from build123d import *

# Parameters (mm, degrees)
F0_W     = 1905
F0_H     = 101.6
F1_DEPTH = 25.4
F3_DEPTH = 25.401


with BuildPart() as f1:
    # F0 (on Right) → F1 (new body)
    with BuildSketch(Plane.YZ):
        with Locations((952.5, 50.8)):
            Rectangle(F0_W, F0_H)
    extrude(amount=F1_DEPTH)

    # F2 (on face) → F3 (cut, through all)
    with BuildSketch(Plane.YZ.offset(25.4)):
        with BuildLine():
            ThreePointArc((63.5, 76.2), (59.780256, 85.180256), (50.8, 88.9))
            Line((50.8, 88.9), (50.8, 63.5))
            ThreePointArc((50.8, 63.5), (59.780256, 67.219744), (63.5, 76.2))
        make_face()
        with BuildLine():
            Line((50.8, 63.5), (50.8, 88.9))
            ThreePointArc((50.8, 88.9), (38.1, 76.2), (50.8, 63.5))
        make_face()
        with BuildLine():
            ThreePointArc((1866.9, 76.2), (1863.180256, 85.180256), (1854.2, 88.9))
            Line((1854.2, 88.9), (1854.2, 63.5))
            ThreePointArc((1854.2, 63.5), (1863.180256, 67.219744), (1866.9, 76.2))
        make_face()
        with BuildLine():
            Line((1854.2, 63.5), (1854.2, 88.9))
            ThreePointArc((1854.2, 88.9), (1841.5, 76.2), (1854.2, 63.5))
        make_face()
    extrude(amount=-F3_DEPTH, mode=Mode.SUBTRACT)


solid = f1.part
For this review, take the finished solid that the model builds, in its own axes (mm). Round coordinates to 2 decimals unless told otherwise and drop trailing zeros. Write item = value, one per line. Start each with the question number.
1. Wall thickness on L1, parallel to Y at x = 14, z = 71; L2, parallel to Y at x = 24.25, z = 85: over which ranges is each line inside the solid? List them lowest first.
2. For pin 1 Ø8 at (y, z) = (1378, 64) entering from -X, flat-tipped, find the tip position at first contact; note if it passes through.
3. Draft analysis for pull direction X (two halves, no side actions). For faces 1 (the face through (25.4, 939, 52)), 2 (the face through (0, 939, 52)), state which applies: released by +X, released by -X, zero draft, split by the parting line, or undercut.
Evaluation:
q1.L1 = 0 to 39.21, 62.39 to 1842.61, 1865.79 to 1905
q1.L2 = 0 to 41.64, 59.96 to 1845.04, 1863.36 to 1905
q2.pin_1 = 0
q3.face_1 = released by +X
q3.face_2 = released by -X
